Check sheet for the modelled part. Datum: model origin and axes. Units: mm. Round coordinates to 2 decimals unless told otherwise and drop trailing zeros. Loops run counter-clockwise (first coordinate to the right, second up) from the corner with the lowest first, then second, coordinate; pieces in that order, holes last. Notation, with made-up numbers: (-2.5, -37) -> (25.5, -37) arc R5 ccw to (25.5, -30) -> close; hole circle Ø10 at (-36, -38.75). An arc over 180 degrees is marked (long way). Use one line per item in the form item = value. Start each with the question number.
(1) Sectioned sample at B-B (x = 5). Record the cut outline in (y, z).
(2) Draft check along X on faces 1 (the cylindrical face through (13.83, 0.06, 6.65)), 2 (the flat face through (17, -2, 5)), 3 (the cylindrical face through (-10.65, -2.97, 4.93)), 4 (the flat face through (-17, -2, 5)). Enter one of: released by +X, released by -X, zero draft, split by the parting line, or undercut.
(3) Sectioned sample at D-D (y = 1.25). State how many separate pieces and enclosed holes the cut face has, and give its area (3 significant figures).
(4) Sectioned sample at A-A (y = 4.25). Record the cut outline in (x, z).
(5) Sectioned sample at C-C (z = 8.75). Record the cut outline in (x, y), and give its area (3 significant figures).
(6) Material ranges on probe 1 along Y at (x, z) = (12.25, 5); probe 2 along X at (y, z) = (-2.25, 5.75); probe 3 along X at (y, z) = (-0.5, 9.25), recorded low to high. Write a range as [from, to].
from build123d import *

# Parameters (mm, degrees)
SKETCH_3_W         = 34
SKETCH_3_H         = 10
EXTRUDE_2_DEPTH    = 10
HOLE_WIZARD_M4_1_D = 3.3
HOLE_WIZARD_M4_2_D = 3.3
HOLE_WIZARD_M4_3_D = 3.3
HOLE_WIZARD_M4_4_D = 3.3
HOLE_WIZARD_M4_5_D = 3.3


with BuildPart() as part:
    # 草图3 → 凸台-拉伸2 (new body)
    with BuildSketch(Plane.XY):
        Rectangle(SKETCH_3_W, SKETCH_3_H)
    extrude(amount=EXTRUDE_2_DEPTH)

    # M4 螺纹孔的螺纹孔钻头1 (through all)
    with Locations(Plane(origin=(17, 0.134296894, 5), x_dir=(0, 0, 1), z_dir=(1, 0, 0))):
        with Locations((0, 0)):
            Hole(HOLE_WIZARD_M4_1_D / 2)

    # M4 螺纹孔的螺纹孔钻头2 (through all)
    with Locations(Plane(origin=(9, -5, 5), x_dir=(-1, 0, 0), z_dir=(0, -1, 0))):
        with Locations((0, 0)):
            Hole(HOLE_WIZARD_M4_2_D / 2)

    # M4 螺纹孔的螺纹孔钻头3 (through all)
    with Locations(Plane(origin=(-9, -5, 5), x_dir=(-1, 0, 0), z_dir=(0, -1, 0))):
        with Locations((0, 0)):
            Hole(HOLE_WIZARD_M4_3_D / 2)

    # M4 螺纹孔的螺纹孔钻头4 (through all)
    with Locations(Plane(origin=(4, 0.134296894, 0), x_dir=(-1, 0, 0), z_dir=(0, 0, -1))):
        with Locations((0, 0)):
            Hole(HOLE_WIZARD_M4_4_D / 2)

    # M4 螺纹孔的螺纹孔钻头5 (through all)
    with Locations(Plane(origin=(-4, 0, 0), x_dir=(-1, 0, 0), z_dir=(0, 0, -1))):
        with Locations((0, 0)):
            Hole(HOLE_WIZARD_M4_5_D / 2)


solid = part.part
Checks:
q1.outline = (-5, 0) -> (-1.18, 0) -> (-1.18, 4) arc R1.65 cw to (-1.18, 6) -> (-1.18, 10) -> (-5, 10) -> close; (1.45, 0) -> (5, 0) -> (5, 10) -> (1.45, 10) -> (1.45, 6) arc R1.65 cw to (1.45, 4) -> close
q2.face_1 = zero draft
q2.face_2 = released by +X
q2.face_3 = undercut
q2.face_4 = released by -X
q3.separate_pieces = 6
q3.enclosed_holes = 0
q3.area = 220 mm2
q4.outline = (-17, 0) -> (17, 0) -> (17, 10) -> (-17, 10) -> close; hole circle Ø3.3 at (-9, 5); hole circle Ø3.3 at (9, 5)
q5.outline = (-17, -5) -> (17, -5) -> (17, 5) -> (-17, 5) -> close; hole circle Ø3.3 at (-4, 0); hole circle Ø3.3 at (4, 0.13)
q5.area = 323 mm2
q6.probe_1 = [-5, -1.52], [1.78, 5]
q6.probe_2 = [-17, -10.47], [-7.53, 7.53], [10.47, 17]
q6.probe_3 = [-17, -5.57], [-2.43, 2.48], [5.52, 17]
